from build123d import *

# Parameters (mm, degrees)
SKETCH_1_W          = 60
SKETCH_1_H          = 30
EXTRUDE_1_DEPTH     = 30
SKETCH_2_W          = 60
SKETCH_2_H          = 30
CUT_EXTRUDE_1_DEPTH = 27
SKETCH_3_R          = 1.6
SKETCH_3_R_2        = 14.1
CUT_EXTRUDE_2_DEPTH = 43.532340636
SKETCH_4_W          = 80
SKETCH_4_H          = 50
SKETCH_4_W_2        = 60
SKETCH_4_H_2        = 30
EXTRUDE_2_DEPTH     = 3
SKETCH_5_R          = 1.6
CUT_EXTRUDE_3_DEPTH = 3
FILLET_1_R          = 3


with BuildPart() as part:
    # 草图1 → 凸台-拉伸1 (new body)
    with BuildSketch(Plane.XY):
        Rectangle(SKETCH_1_W, SKETCH_1_H)
    extrude(amount=EXTRUDE_1_DEPTH)

    # 草图2 → 切除-拉伸1 (cut)
    with BuildSketch(Plane.XZ.offset(15)):
        with Locations((0, 15)):
            Rectangle(SKETCH_2_W, SKETCH_2_H)
    extrude(amount=-CUT_EXTRUDE_1_DEPTH, mode=Mode.SUBTRACT)

    # 草图3 → 切除-拉伸2 (cut, through all)
    with BuildSketch(Plane(origin=(0, 15, 0), x_dir=(1, 0, 0), z_dir=(0, 1, 0))):
        with Locations(Location((-27.02081528, -2.97918472, 0), (0, 0, 270))):
            Circle(SKETCH_3_R)
        with Locations(Location((-2.97918472, -2.97918472, 0), (0, 0, 270))):
            Circle(SKETCH_3_R)
        with Locations(Location((-2.97918472, -27.02081528, 0), (0, 0, 270))):
            Circle(SKETCH_3_R)
        with Locations(Location((-27.02081528, -27.02081528, 0), (0, 0, 270))):
            Circle(SKETCH_3_R)
        with Locations(Location((27.02081528, -27.02081528, 0), (0, 0, 90))):
            Circle(SKETCH_3_R)
        with Locations(Location((2.97918472, -27.02081528, 0), (0, 0, 90))):
            Circle(SKETCH_3_R)
        with Locations(Location((2.97918472, -2.97918472, 0), (0, 0, 90))):
            Circle(SKETCH_3_R)
        with Locations(Location((27.02081528, -2.97918472, 0), (0, 0, 90))):
            Circle(SKETCH_3_R)
        with Locations(Location((-15, -15, 0), (0, 0, 270))):
            Circle(SKETCH_3_R_2)
        with Locations(Location((15, -15, 0), (0, 0, 270))):
            Circle(SKETCH_3_R_2)
    extrude(amount=-CUT_EXTRUDE_2_DEPTH, mode=Mode.SUBTRACT)

    # 草图4 → 凸台-拉伸2 (add)
    with BuildSketch(Plane(origin=(0, 15, 0), x_dir=(1, 0, 0), z_dir=(0, 1, 0))):
        with Locations((0, -15)):
            Rectangle(SKETCH_4_W, SKETCH_4_H)
        with Locations((0, -15)):
            Rectangle(SKETCH_4_W_2, SKETCH_4_H_2, mode=Mode.SUBTRACT)
    extrude(amount=-EXTRUDE_2_DEPTH)

    # 草图5 → 切除-拉伸3 (cut)
    with BuildSketch(Plane(origin=(0, 15, 0), x_dir=(1, 0, 0), z_dir=(0, 1, 0))):
        with Locations(Location((-35, 5, 0), (0, 0, 270))):
            Circle(SKETCH_5_R)
        with Locations(Location((35, 5, 0), (0, 0, 270))):
            Circle(SKETCH_5_R)
        with Locations(Location((35, -35, 0), (0, 0, 270))):
            Circle(SKETCH_5_R)
        with Locations(Location((-35, -35, 0), (0, 0, 270))):
            Circle(SKETCH_5_R)
    extrude(amount=-CUT_EXTRUDE_3_DEPTH, mode=Mode.SUBTRACT)

    # 圆角1
    fillet_1_edges = [part.edges().sort_by_distance(p)[0] for p in [
        (40, 13.5, -10),
        (40, 13.5, 40),
        (-40, 13.5, 40),
        (-40, 13.5, -10),
    ]]
    fillet(fillet_1_edges, radius=FILLET_1_R)


solid = part.part
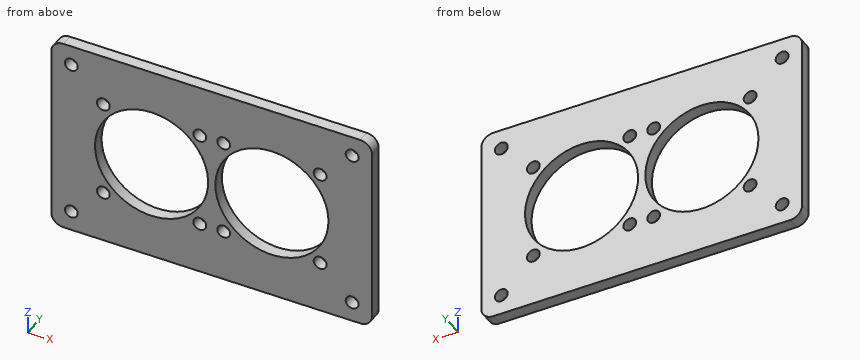
The model under review builds one solid part; all positions refer to its coordinate system, in mm. Coordinates: 2 decimals unless noted, no trailing zeros. Loops run counter-clockwise (first coordinate to the right, second up) from the corner with the lowest first, then second, coordinate; pieces in that order, holes last.
(1) Consider section A-A, the plane x = -35. Give the boundary of the cut face in (y, z).
Determined:
outline: (12, -10) - (15, -10) - (15, -6.6) - (12, -6.6) - close; (12, -3.4) - (15, -3.4) - (15, 33.4) - (12, 33.4) - close; (12, 36.6) - (15, 36.6) - (15, 40) - (12, 40) - close
(2) Wall thickness on L1, parallel to X at y = 13.3, z = 14.5; L2, parallel to X at y = 12.85, z = 35; L3, parallel to Z at x = 26, y = 13.4: over which ranges is each line inside the solid? List them lowest first.
Determined:
L1: x = -40 to -29.09, -0.91 to 0.91, 29.09 to 40
L2: x = -40 to -36.6, -33.4 to 33.4, 36.6 to 40
L3: z = -10 to 1.75, 4.21 to 6.18, 23.82 to 25.79, 28.25 to 40
(3) Insertion check: P1, Ø1.9, axis at x = 27.02, z = 27.02, coming from the +Y side. The pin has a flat end and moves straight along its axis. Give the tip position at first contact, or say it passes through.
Determined:
P1: passes through
(4) Consider section C-C, the plane x = 10.5. Give the boundary of the cut face in (y, z), plus the area to 3 significant figures.
Determined:
outline: (12, -10) - (15, -10) - (15, 1.64) - (12, 1.64) - close; (12, 28.36) - (15, 28.36) - (15, 40) - (12, 40) - close
area: 69.8 mm2
(5) Consider section D-D, the plane y = 12.95. Give the number of separate pieces and of enclosed holes in the cut face, plus the area to 3 significant figures.
Determined:
separate pieces: 1
enclosed holes: 14
area: 2,650 mm2
(6) Consider section B-B, the plane z = 15. Give the boundary of the cut face in (x, y).
Determined:
outline: (-40, 12) - (-29.1, 12) - (-29.1, 15) - (-40, 15) - close; (-0.9, 12) - (0.9, 12) - (0.9, 15) - (-0.9, 15) - close; (29.1, 12) - (40, 12) - (40, 15) - (29.1, 15) - close
